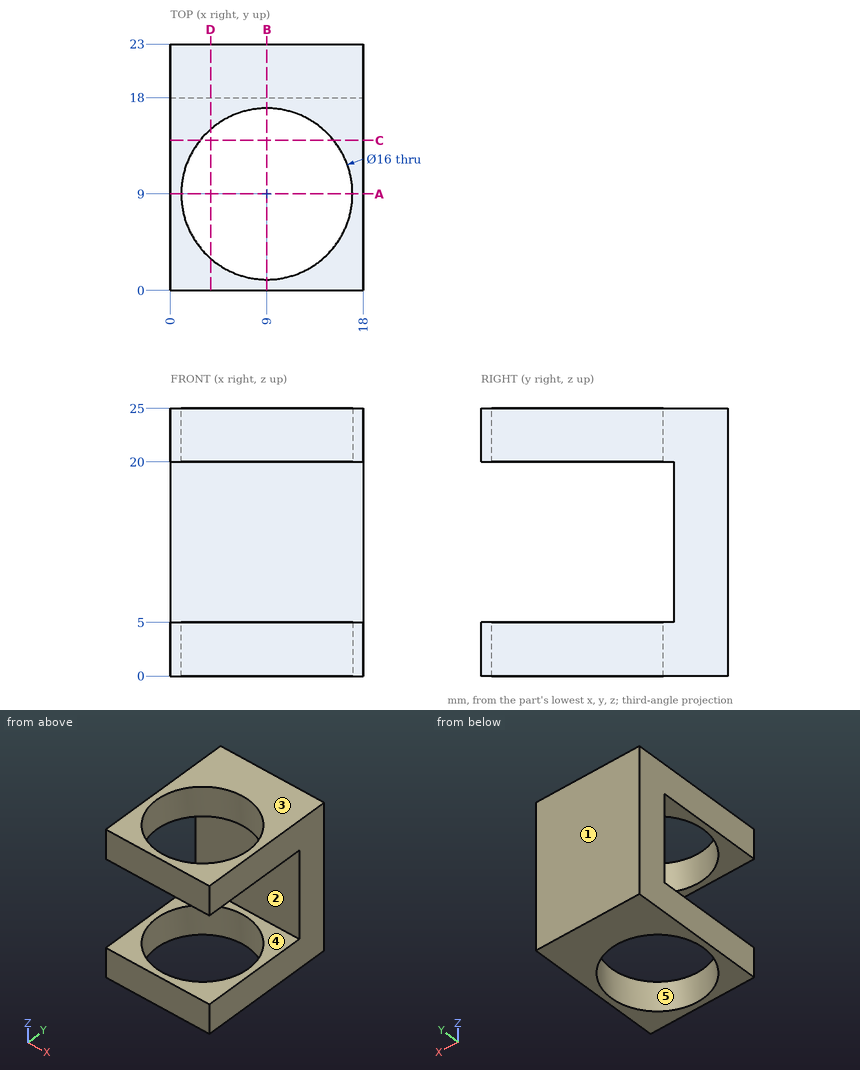
Design review of the part shown in the three views and the two pictorial views. Dimensions are in mm from the part's minimum x, y and z. A direction names the side the tool comes from. Give positions to 0.01 mm unless a question says otherwise; leave off trailing zeros. Write each loop counter-clockwise with the first axis right and the second up, starting at its lowest first coordinate (ties: lowest second). Pieces come first, ordered by that corner, then holes.
(1) Wall thickness on line 1 along Z through (x, y) = (1.25, 5.5); line 2 along Y through (x, z) = (9, 23.8); line 3 along Y through (x, z) = (17.75, 16.25): over which ranges is each line inside the solid? List them lowest first.
Checked values:
line 1: z = 0 to 5, 20 to 25
line 2: y = 0 to 1, 17 to 23
line 3: y = 18 to 23
(2) Add section B-B (x = 9). Give the boundary of the cut face in (y, z), and give its area (3 significant figures).
Checked values:
outline: (0, 0) - (1, 0) - (1, 5) - (0, 5) - close; (0, 20) - (1, 20) - (1, 25) - (0, 25) - close; (17, 0) - (23, 0) - (23, 25) - (17, 25) - (17, 20) - (18, 20) - (18, 5) - (17, 5) - close
area: 145 mm2
(3) Add section C-C (y = 14). Give the boundary of the cut face in (x, z) (3 decimals).
Checked values:
outline: (0, 0) - (2.755, 0) - (2.755, 5) - (0, 5) - close; (0, 20) - (2.755, 20) - (2.755, 25) - (0, 25) - close; (15.245, 0) - (18, 0) - (18, 5) - (15.245, 5) - close; (15.245, 20) - (18, 20) - (18, 25) - (15.245, 25) - close
(4) Tool access review of the marked faces 4 and 5: name each direction out of +Z, -Z, +X, -X, +Y, -Y from which nothing blocks a thin tool from reaching the whole face with its end or side.
Checked values:
face 4: +X, -X, -Y
face 5: +Z, -Z
(5) Mouldability with a two-part tool opening along Z and no side actions: class the marked faces 1, 2 and 3 as +Z half, -Z half, draft (parallel to the pull), parting line (faces both ways), or undercut.
Checked values:
face 1: draft
face 2: undercut
face 3: +Z half
(6) Clearance check with a flat-ended pin moving along its axis: pin 1 Ø3 at (x, z) = (7.5, 11.5) entering from -Y. State where the tip first meets the part, or that it passes through.
Checked values:
pin 1: stops at y = 18
(7) Add section D-D (x = 3.75). Give the boundary of the cut face in (y, z).
Checked values:
outline: (0, 0) - (2.96, 0) - (2.96, 5) - (0, 5) - close; (0, 20) - (2.96, 20) - (2.96, 25) - (0, 25) - close; (15.04, 0) - (23, 0) - (23, 25) - (15.04, 25) - (15.04, 20) - (18, 20) - (18, 5) - (15.04, 5) - close
(8) Add section A-A (y = 9). Give the boundary of the cut face in (x, z).
Checked values:
outline: (0, 0) - (1, 0) - (1, 5) - (0, 5) - close; (0, 20) - (1, 20) - (1, 25) - (0, 25) - close; (17, 0) - (18, 0) - (18, 5) - (17, 5) - close; (17, 20) - (18, 20) - (18, 25) - (17, 25) - close
